```python
from build123d import *

# Parameters (mm, degrees)
EXTRUDE_1_DEPTH             = 40
SKETCH_8_R                  = 1.5
CUT_EXTRUDE_2_DEPTH         = 96.336247042
SKETCH_12_W                 = 30
SKETCH_12_H                 = 40
SKETCH_12_R                 = 1.5
EXTRUDE_7_DEPTH             = 66.5
EXTRUDE_7_DIRECTION_2_REACH = 97.336
CUT_EXTRUDE_3_DEPTH         = 112.45514793
CUT_EXTRUDE_START           = -50
SKETCH_15_R                 = 3.5
CUT_EXTRUDE_4_DEPTH         = 84.791815893
EXTRUDE_START               = -58.6
SKETCH_16_W                 = 6
SKETCH_16_H                 = 21
EXTRUDE_9_DEPTH             = 58.6
SKETCH_17_R                 = 2
CUT_EXTRUDE_5_DEPTH         = 112.45514793


with BuildPart() as part:
    # 草图1 → 凸台-拉伸1 (new body)
    with BuildSketch(Plane(origin=(0, 0, 0), x_dir=(1, 0, 0), z_dir=(0, 1, 0))):
        Polygon((0, 0), (80, 0), (80, 6), (20, 6), (20, 27), (80, 27), (80, 33), (0, 33), align=None)
    extrude(amount=EXTRUDE_1_DEPTH)

    # 草图8 → 切除-拉伸2 (cut, through all)
    with BuildSketch(Plane(origin=(0, 0, -33), x_dir=(-1, 0, 0), z_dir=(0, 0, -1))):
        with Locations((-74, 8)):
            Circle(SKETCH_8_R)
        with Locations((-74, 32)):
            Circle(SKETCH_8_R)
        with Locations((-6, 32)):
            Circle(SKETCH_8_R)
        with Locations((-6, 8)):
            Circle(SKETCH_8_R)
    extrude(amount=-CUT_EXTRUDE_2_DEPTH, mode=Mode.SUBTRACT)

    # 草图12 → 凸台-拉伸7 (add)
    with BuildSketch(Plane.XY):
        with Locations((-5, 20)):
            Rectangle(SKETCH_12_W, SKETCH_12_H)
        with Locations((-11, 32)):
            Circle(SKETCH_12_R, mode=Mode.SUBTRACT)
        with Locations((-11, 8)):
            Circle(SKETCH_12_R, mode=Mode.SUBTRACT)
        with Locations(Location((6, 8, 0), (0, 0, 180))):
            Circle(SKETCH_12_R, mode=Mode.SUBTRACT)
        with Locations(Location((6, 32, 0), (0, 0, 180))):
            Circle(SKETCH_12_R, mode=Mode.SUBTRACT)
    extrude(amount=EXTRUDE_7_DEPTH)

    # 凸台-拉伸7 direction 2: up to this face of the body (flat: up to its plane)
    extrude_7_direction_2_end = Plane(part.part.faces().sort_by_distance((40, 20, -33))[0])
    # 草图12 → 凸台-拉伸7 direction 2 (add, up to the picked face)
    with BuildSketch(Plane.XY, mode=Mode.PRIVATE) as extrude_7_direction_2_sk1:
        with Locations((-5, 20)):
            Rectangle(SKETCH_12_W, SKETCH_12_H)
        with Locations((-11, 32)):
            Circle(SKETCH_12_R, mode=Mode.SUBTRACT)
        with Locations((-11, 8)):
            Circle(SKETCH_12_R, mode=Mode.SUBTRACT)
        with Locations(Location((6, 8, 0), (0, 0, 180))):
            Circle(SKETCH_12_R, mode=Mode.SUBTRACT)
        with Locations(Location((6, 32, 0), (0, 0, 180))):
            Circle(SKETCH_12_R, mode=Mode.SUBTRACT)
    extrude_7_direction_2_tool1 = split(extrude(extrude_7_direction_2_sk1.sketch, amount=-EXTRUDE_7_DIRECTION_2_REACH, mode=Mode.PRIVATE), bisect_by=extrude_7_direction_2_end, keep=Keep.BOTH, mode=Mode.PRIVATE)
    add(extrude_7_direction_2_tool1.solids().sort_by(Axis((-5.060326, 20, 0), (0, 0, -1)))[0])

    # 草图14 → 切除-拉伸3 (cut, through all)
    with BuildSketch(Plane(origin=(0, 40, 0), x_dir=(1, 0, 0), z_dir=(0, 1, 0))):
        Polygon((-20, 33), (0, 33), (-20, 13), align=None)
    extrude(amount=-CUT_EXTRUDE_3_DEPTH, mode=Mode.SUBTRACT)

    # 草图15 → 切除-拉伸4 (cut, through all)
    with BuildSketch(Plane.XY.offset(66.5).offset(CUT_EXTRUDE_START)):
        with Locations((-11, 32)):
            Circle(SKETCH_15_R)
        with Locations((-11, 8)):
            Circle(SKETCH_15_R)
    extrude(amount=-CUT_EXTRUDE_4_DEPTH, mode=Mode.SUBTRACT)

    # 草图16 → 凸台-拉伸9 (add)
    with BuildSketch(Plane(origin=(0, 40, 0), x_dir=(1, 0, 0), z_dir=(0, 1, 0)).offset(EXTRUDE_START)):
        with Locations((65, 16.5)):
            Rectangle(SKETCH_16_W, SKETCH_16_H)
    extrude(amount=EXTRUDE_9_DEPTH)

    # 草图17 → 切除-拉伸5 (cut, through all)
    with BuildSketch(Plane.XY):
        with Locations((32, 15)):
            Circle(SKETCH_17_R)
    extrude(amount=-CUT_EXTRUDE_5_DEPTH, mode=Mode.SUBTRACT)


solid = part.part
```
For this review, take the finished solid that the model builds, in its own axes (mm). A direction names the side the tool comes from. Round coordinates to 2 decimals unless told otherwise and drop trailing zeros. Write each loop counter-clockwise with the first axis right and the second up, starting at its lowest first coordinate (ties: lowest second). Pieces come first, ordered by that corner, then holes. Notation, with made-up numbers: (15, 23.5) - (46, 23.5) arc R18 ccw to (46, 27.5) - close; hole circle Ø8 at (-19, 27). An arc over 180 degrees is marked (long way). Put each result on its own line as item: value.
Q1. We need section C-C (x = 45). Give the boundary of the cut face in (y, z).
Solved:
outline: (0, -33) - (40, -33) - (40, -27) - (0, -27) - close; (0, -6) - (40, -6) - (40, 0) - (0, 0) - close
Q2. Wall thickness on probe 1 along X at (y, z) = (8, 39.5); probe 2 along Y at (x, z) = (6, 10); probe 3 along Z at (x, y) = (39.5, 16.5): over which ranges is each line inside the solid? List them lowest first.
Solved:
probe 1: x = -20 to -12.5, -9.5 to 4.5, 7.5 to 10
probe 2: y = 0 to 6.5, 9.5 to 30.5, 33.5 to 40
probe 3: z = -33 to -27, -6 to 0
Q3. Machinability: for faces 1 (the face through (65, -9, -27)), 2 (the face through (-11, 6, 16.5)), 3 (the face through (74, 20, -6)), which of the approach directions +Z, -Z, +X, -X, +Y, -Y give a long, thin tool a straight path to every point of the face, cutting with its end or side? Answer none if there is none.
Solved:
face 1: -Z, +X, -X, -Y
face 2: -Z
face 3: +X, +Y, -Y
Q4. We need section D-D (x = -11). Give the boundary of the cut face in (y, z).
Solved:
outline: (0, -22) - (4.5, -22) - (4.5, 16.5) - (6.5, 16.5) - (6.5, 66.5) - (0, 66.5) - close; (9.5, 16.5) - (11.5, 16.5) - (11.5, -22) - (28.5, -22) - (28.5, 16.5) - (30.5, 16.5) - (30.5, 66.5) - (9.5, 66.5) - close; (33.5, 16.5) - (35.5, 16.5) - (35.5, -22) - (40, -22) - (40, 66.5) - (33.5, 66.5) - close
Q5. We need section A-A (x = 74). Give the boundary of the cut face in (y, z).
Solved:
outline: (0, -33) - (6.5, -33) - (6.5, -27) - (0, -27) - close; (0, -6) - (6.5, -6) - (6.5, 0) - (0, 0) - close; (9.5, -33) - (30.5, -33) - (30.5, -27) - (9.5, -27) - close; (9.5, -6) - (30.5, -6) - (30.5, 0) - (9.5, 0) - close; (33.5, -33) - (40, -33) - (40, -27) - (33.5, -27) - close; (33.5, -6) - (40, -6) - (40, 0) - (33.5, 0) - close
Q6. We need section B-B (y = 20). Give the boundary of the cut face in (x, z), and give its area (3 significant figures).
Solved:
outline: (-20, -13) - (0, -33) - (80, -33) - (80, -27) - (68, -27) - (68, -6) - (80, -6) - (80, 0) - (10, 0) - (10, 66.5) - (-20, 66.5) - close; hole (20, -27) - (62, -27) - (62, -6) - (20, -6) - close
area: 3,960 mm2
Q7. Mouldability with a two-part tool opening along Z and no side actions: class faces 4 (the face through (62, 10, -16)), 5 (the face through (65, -9, -6)), 6 (the face through (-11.325, 30.536, 41.15)) as released by +Z, released by -Z, zero draft, split by the parting line, or undercut.
Solved:
face 4: undercut
face 5: released by +Z
face 6: zero draft
Q8. Insertion check: pin 1 Ø2.5 at (x, y) = (6, 8) entering from +Z; pin 2 Ø1.5 at (y, z) = (19.5, 44.5) entering from +X; pin 3 Ø10.5 at (y, z) = (24.5, -17) entering from +X; pin 4 Ø12 at (x, y) = (61.5, -8) entering from -Z. Each pin has a flat end and moves straight along its axis. Give the tip position at first contact, or say it passes through.
Solved:
pin 1: passes through
pin 2: stops at x = 10
pin 3: stops at x = 68
pin 4: stops at z = -27
